Model file for the job. Use its own axes, mm. A direction names the side the tool comes from. Round coordinates to 2 decimals unless told otherwise and drop trailing zeros. Order: outer loops, then holes, each group sorted by start corner. A loop starts at its lowest first (then second) coordinate and runs counter-clockwise, first axis right, second up. Notation, with made-up numbers: (54, -23.5) - (62, -23.5) arc R16 ccw to (62, -4.5) - close; hole circle Ø8 at (45.5, 84). An arc over 180 degrees is marked (long way). Put each result on its own line as item: value. Start each with the question number.
Item 1: Which spindle directions (+Z, -Z, +X, -X, +Y, -Y) get a long thin tool onto all of the face, cutting with end or side? Do faces 1 (the face through (-1, -25.4, 9)), 2 (the face through (-52, -8, 5.842)). Say none if no direction does.
Item 2: Saw through at A-A on x = -46.5. List the corners of the cut face in (y, z), plus the area to 3 significant figures.
Item 3: Saw through at B-B on y = 3.5. List the corners of the cut face in (x, z).
Item 4: Mould opens along Y. For faces 3 (the face through (1, 25.4, 9)), 4 (the face through (76.2, 0, 9)), 5 (the face through (38.68, -1.11, 12.41)), 6 (the face through (49.1, -8.5, 5.588)) say: pulls with the +Y half, pulls with the -Y half, needs draft (parallel to the pull), parting line crosses it, or undercut.
Item 5: Probe probe 1 along X at (y, z) = (3.5, 13.25); probe 2 along X at (y, z) = (-8, 13.25); probe 3 along Y at (x, z) = (43, 12.75). List the from-to ranges inside material, lowest first.
Item 6: Saw through at D-D on x = 52. List the corners of the cut face in (y, z), plus the area to 3 significant figures.
Item 7: Saw through at C-C on z = 13.25. List the corners of the cut face in (x, y).
Item 8: Pin check, flat tip, straight feed: pin 1 Ø1.5 at (x, y) = (-56, 0) entering from +Z. Stop position of the tip, or through.
```python
from build123d import *

# Parameters (mm, degrees)
F0_R     = 6.731
F1_DEPTH = 19.05
F2_R     = 9.906
F2_R_2   = 6.731
F3_DEPTH = 13.208
F4_R     = 10.541
F4_R_2   = 6.731
F5_DEPTH = 13.462


with BuildPart() as f1:
    # F0 (on Top) → F1 (new body)
    with BuildSketch(Plane.XY):
        Polygon((22.225, -25.4), (76.2, -25.4), (76.2, 25.4), (-76.2, 25.4), (-76.2, -25.4), align=None)
        with Locations((-49.2125, -1.5748)):
            Circle(F0_R, mode=Mode.SUBTRACT)
        with Locations((49.2125, -1.5748)):
            Circle(F0_R, mode=Mode.SUBTRACT)
    extrude(amount=F1_DEPTH)

    # F2 (on face) → F3 (cut)
    with BuildSketch(Plane.XY.offset(19.05)):
        with Locations((-49.2125, -1.5748)):
            Circle(F2_R)
        with Locations((-49.2125, -1.5748)):
            Circle(F2_R_2, mode=Mode.SUBTRACT)
    extrude(amount=-F3_DEPTH, mode=Mode.SUBTRACT)

    # F4 (on face) → F5 (cut)
    with BuildSketch(Plane.XY.offset(19.05)):
        with Locations((49.2125, -1.5748)):
            Circle(F4_R)
        with Locations((49.2125, -1.5748)):
            Circle(F4_R_2, mode=Mode.SUBTRACT)
    extrude(amount=-F5_DEPTH, mode=Mode.SUBTRACT)


solid = f1.part
```
Results found:
1. face 1: +Z, -Z, +X, -X, -Y
1. face 2: +Z
2. outline: (-25.4, 0) - (-7.74, 0) - (-7.74, 5.84) - (-11.1, 5.84) - (-11.1, 19.05) - (-25.4, 19.05) - close; (4.59, 0) - (25.4, 0) - (25.4, 19.05) - (7.95, 19.05) - (7.95, 5.84) - (4.59, 5.84) - close
2. area: 644 mm²
3. outline: (-76.2, 0) - (-53.63, 0) - (-53.63, 5.84) - (-57.72, 5.84) - (-57.72, 19.05) - (-76.2, 19.05) - close; (-44.79, 0) - (44.79, 0) - (44.79, 5.59) - (39.97, 5.59) - (39.97, 19.05) - (-40.71, 19.05) - (-40.71, 5.84) - (-44.79, 5.84) - close; (53.63, 0) - (76.2, 0) - (76.2, 19.05) - (58.45, 19.05) - (58.45, 5.59) - (53.63, 5.59) - close
4. face 3: pulls with the +Y half
4. face 4: needs draft
4. face 5: undercut
4. face 6: undercut
5. probe 1: x = -76.2 to -57.72, -40.71 to 39.97, 58.45 to 76.2
5. probe 2: x = -76.2 to -56.75, -41.67 to 40.86, 57.57 to 76.2
5. probe 3: y = -25.4 to -10.09, 6.94 to 25.4
6. outline: (-25.4, 0) - (-7.7, 0) - (-7.7, 5.59) - (-11.74, 5.59) - (-11.74, 19.05) - (-25.4, 19.05) - close; (4.55, 0) - (25.4, 0) - (25.4, 19.05) - (8.59, 19.05) - (8.59, 5.59) - (4.55, 5.59) - close
6. area: 626 mm²
7. outline: (-76.2, -25.4) - (76.2, -25.4) - (76.2, 25.4) - (-76.2, 25.4) - close; hole circle Ø19.81 at (-49.21, -1.57); hole circle Ø21.08 at (49.21, -1.57)
8. pin 1: stops at z = 5.84
